Could you check a few things on this model? Use its own coordinates, in mm. A direction names the side the tool comes from. Round coordinates to 2 decimals unless told otherwise and drop trailing zeros. Loops run counter-clockwise (first coordinate to the right, second up) from the corner with the lowest first, then second, coordinate; pieces in that order, holes last.
from build123d import *

# Parameters (mm, degrees)
BOSS_EXTRUDE1_DEPTH      = 3
BOSS_EXTRUDE2_DEPTH      = 4
CUT_EXTRUDE4_DEPTH       = 3
CUT_EXTRUDE5_DEPTH       = 3
BOSS_EXTRUDE3_DEPTH      = 5
BOSS_EXTRUDE3_DEPTH_BACK = 1
SKETCH7_W                = 2
SKETCH7_H                = 1
BOSS_EXTRUDE4_DEPTH      = 5


with BuildPart() as part:
    # Sketch2 → Boss-Extrude1 (new body)
    with BuildSketch(Plane(origin=(0, 0, 0), x_dir=(1, 0, 0), z_dir=(0, 1, 0))):
        Polygon((0, 0), (2, 0), (5, -5), (7, -5), (7, 2), (5, 2), (5, 0), (3, 0), (3, 2), (0, 2), align=None)
    extrude(amount=BOSS_EXTRUDE1_DEPTH)

    # Sketch3 → Boss-Extrude2 (add)
    with BuildSketch(Plane(origin=(0, 3, 0), x_dir=(1, 0, 0), z_dir=(0, 1, 0))):
        Polygon((3, 0), (3, 1), (0, 1), (0, 0), (2, 0), (5, -5), (7, -5), (7, 1), (5, 1), (5, 0), align=None)
        Polygon((2, 0), (0, 0), (0, -5), (5, -5), align=None)
    extrude(amount=BOSS_EXTRUDE2_DEPTH)

    # Sketch5 → Cut-Extrude4 (cut)
    with BuildSketch(Plane.ZY.offset(-5)):
        Polygon((5, 4), (5, 7), (2, 7), align=None)
    extrude(amount=CUT_EXTRUDE4_DEPTH, mode=Mode.SUBTRACT)

    # 3DSketch1 → Cut-Extrude5 (cut, along a direction that is not the sketch's normal)
    with BuildSketch(Plane(origin=(0, 5, 5), x_dir=(0, 0.7071067811865476, -0.7071067811865476), z_dir=(0.5773502691896267, -0.5773502691896254, -0.5773502691896254))):
        Polygon((0, 0), (1.414213562, 2.449489743), (2.828427125, 0), align=None)
    extrude(amount=-CUT_EXTRUDE5_DEPTH, dir=(1, 0, 0), mode=Mode.SUBTRACT)

    # Sketch6 → Boss-Extrude3 (add, two sides)
    with BuildSketch(Plane.XY) as boss_extrude3_sk:
        Polygon((7, 7), (10, 5), (10, 2), (7, 2), align=None)
    extrude(amount=BOSS_EXTRUDE3_DEPTH)
    extrude(boss_extrude3_sk.sketch, amount=-BOSS_EXTRUDE3_DEPTH_BACK)

    # Sketch7 → Boss-Extrude4 (add)
    with BuildSketch(Plane(origin=(0, 7, 0), x_dir=(1, 0, 0), z_dir=(0, 1, 0))):
        with Locations((8, -1.5)):
            Rectangle(SKETCH7_W, SKETCH7_H)
    extrude(amount=-BOSS_EXTRUDE4_DEPTH)


solid = part.part
Item 1: If we section it at D-D, the plane x = 7.5: Please give me the cut outline in (y, z), then the cut area to 3 significant figures.
Results list:
outline: (2, -1) - (6.67, -1) - (6.67, 1) - (7, 1) - (7, 2) - (6.67, 2) - (6.67, 5) - (2, 5) - close
area: 28.3 mm2
Item 2: If we section it at B-B, the plane y = 1.25: Please give me the cut outline in (x, z).
Results list:
outline: (0, -2) - (3, -2) - (3, 0) - (5, 0) - (5, -2) - (7, -2) - (7, 5) - (5, 5) - (2, 0) - (0, 0) - close
Item 3: Will these pins go through, and if not, where does the flat tip stop? pin 1 (0.8 mm diameter, centred on y = 6.5, z = 1.5, fed in from +X); pin 2 (0.5 mm diameter, centred on x = 6, z = -1.5, fed in from +Y); pin 3 (2.5 mm diameter, centred on x = 6.5, y = 4.5, fed in from -Z).
Results list:
pin 1: stops at x = 9
pin 2: stops at y = 3
pin 3: stops at z = -1
Item 4: We'd pull the mould along X, two halves only. Please class faces 5 (the flat face through (2, 6, 4)), 6 (the flat face through (4, 3, 0)), 7 (the flat face through (8.4, 6.6, 1)), 8 (the flat face through (10, 4, 2)): released by +X, released by -X, zero draft, split by the parting line, or undercut.
Results list:
face 5: undercut
face 6: undercut
face 7: zero draft
face 8: released by +X
Item 5: If we section it at C-C, the plane z = 4.5: Please give me the cut outline in (x, y).
Results list:
outline: (0, 3) - (4.7, 3) - (4.7, 0) - (7, 0) - (7, 2) - (10, 2) - (10, 5) - (7, 7) - (5, 7) - (5, 4.5) - (2, 4.5) - (2, 7) - (1.5, 7) - (0, 5.5) - close
Item 6: For faces 1 (the flat face through (5, 2.7, -0.8)), 2 (the flat face through (1, 1, 0)), 3 (the flat face through (2, 5, -1)), 4 (the flat face through (5, 6, 4)), which set-ups out of +Z, -Z, +X, -X, +Y, -Y let a thin tool reach every point of the face, with its end or its side?
Results list:
face 1: -Z, +Y, -Y
face 2: +Z, -X, -Y
face 3: -Z, +X, -X, +Y
face 4: +Z, +Y
Item 7: If we section it at A-A, the plane z = -0.25: Please give me the cut outline in (x, y), then the cut area to 3 significant figures.
Results list:
outline: (0, 0) - (3, 0) - (3, 7) - (0, 7) - close; (5, 0) - (7, 0) - (7, 2) - (10, 2) - (10, 5) - (7, 7) - (5, 7) - close
area: 47.0 mm2
Item 8: If I drill on line 1 along X through (y, z) = (2.5, -0.25); line 2 along Y through (x, z) = (5.5, -1.25); line 3 along Z through (x, y) = (6.5, 6.25), over which ranges is the centre line in solid material (lowest first)?
Results list:
line 1: x = 0 to 3, 5 to 10
line 2: y = 0 to 3
line 3: z = -1 to 5
